from build123d import *

# Parameters (mm, degrees)
SKETCH_W        = 65
SKETCH_H        = 42
PAD_DEPTH       = 4.5
SKETCH001_W     = 2
SKETCH001_H     = 2
POCKET_DEPTH    = 1.5
SKETCH002_W     = 2
SKETCH002_H     = 3
POCKET001_DEPTH = 0.8
SKETCH003_W     = 59
SKETCH003_H     = 35
POCKET002_DEPTH = 3.9
SKETCH004_W     = 2
SKETCH004_H     = 0.4
POCKET003_DEPTH = 5


with BuildPart() as part:
    # Sketch → Pad (new body)
    with BuildSketch(Plane.XY):
        with Locations((-32.5, 0)):
            Rectangle(SKETCH_W, SKETCH_H)
    extrude(amount=-PAD_DEPTH)

    # Sketch001 → Pocket (cut)
    with BuildSketch(Plane.YZ):
        with Locations((-20, -1)):
            Rectangle(SKETCH001_W, SKETCH001_H)
        with Locations((20, -1)):
            Rectangle(SKETCH001_W, SKETCH001_H)
    extrude(amount=-POCKET_DEPTH, mode=Mode.SUBTRACT)

    # Sketch002 → Pocket001 (cut)
    with BuildSketch(Plane.YZ):
        with Locations((-16, -2.2)):
            Rectangle(SKETCH002_W, SKETCH002_H)
        with Locations((-10.8, -2.2)):
            Rectangle(SKETCH002_W, SKETCH002_H)
    extrude(amount=-POCKET001_DEPTH, mode=Mode.SUBTRACT)

    # Sketch003 → Pocket002 (cut)
    with BuildSketch(Plane.XY):
        with Locations((-32.5, 0)):
            Rectangle(SKETCH003_W, SKETCH003_H)
    extrude(amount=-POCKET002_DEPTH, mode=Mode.SUBTRACT)

    # Sketch004 → Pocket003 (cut)
    with BuildSketch(Plane.YZ):
        with Locations((-16, -0.9)):
            Rectangle(SKETCH004_W, SKETCH004_H)
        with Locations((-16, -3.5)):
            Rectangle(SKETCH004_W, SKETCH004_H)
        with Locations((-10.8, -0.9)):
            Rectangle(SKETCH004_W, SKETCH004_H)
        with Locations((-10.8, -3.5)):
            Rectangle(SKETCH004_W, SKETCH004_H)
    extrude(amount=-POCKET003_DEPTH, mode=Mode.SUBTRACT)


solid = part.part
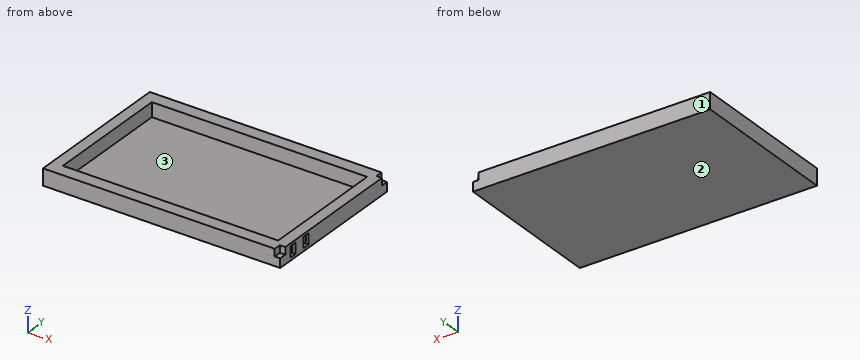
Could you check a few things on this model? Use its own coordinates, in mm. Face numbers are marked on the shaded views. Give positions to 0.01 mm unless a question says otherwise; leave off trailing zeros. Order: outer loops, then holes, each group sorted by start corner. A loop starts at its lowest first (then second) coordinate and runs counter-clockwise, first axis right, second up.
1. Thinking about a two-plate mould opening in Y: for the marked faces 1, 2 and 3, which applies, +Y half, -Y half, draft (parallel to the pull), parting line (faces both ways), or undercut?
Answers below:
face 1: +Y half
face 2: draft
face 3: undercut
2. Suppose I cut it at D-D (y = 10). Write out the boundary of the cut face in (x, z), plus the area to 3 significant figures.
Answers below:
outline: (-65, -4.5) - (0, -4.5) - (0, 0) - (-3, 0) - (-3, -3.9) - (-62, -3.9) - (-62, 0) - (-65, 0) - close
area: 62.4 mm2
3. Suppose I cut it at C-C (x = -35.5). Write out the boundary of the cut face in (y, z), plus the area to 3 significant figures.
Answers below:
outline: (-21, -4.5) - (21, -4.5) - (21, 0) - (17.5, 0) - (17.5, -3.9) - (-17.5, -3.9) - (-17.5, 0) - (-21, 0) - close
area: 52.5 mm2
4. I need wall thicknesses on L1, parallel to X at y = 16, z = -3; L2, parallel to Y at x = -43.5, z = -1.4; L3, parallel to Z at x = -14, y = -16.5. Which ranges of each line are inside material? Lowest first, please.
Answers below:
L1: x = -65 to -62, -3 to 0
L2: y = -21 to -17.5, 17.5 to 21
L3: z = -4.5 to -3.9
5. Suppose I cut it at A-A (z = -2.65). Write out the boundary of the cut face in (x, y), plus the area to 3 significant figures.
Answers below:
outline: (-65, -21) - (0, -21) - (0, -17) - (-0.8, -17) - (-0.8, -15) - (0, -15) - (0, -11.8) - (-0.8, -11.8) - (-0.8, -9.8) - (0, -9.8) - (0, 21) - (-65, 21) - close; hole (-62, -17.5) - (-3, -17.5) - (-3, 17.5) - (-62, 17.5) - close
area: 662 mm2
6. For pin 1 (0.6 mm diameter, centred on y = -16.5, z = -2.5, fed in from +X); pin 2 (1.6 mm diameter, centred on x = -0.5, z = -1, fed in from +Y); pin 3 (5 mm diameter, centred on x = -55.5, y = -11, fed in from +Z), each with a flat end and sliding along its axis, tell me the tip position at first contact or that it passes through.
Answers below:
pin 1: stops at x = -0.8
pin 2: stops at y = 19
pin 3: stops at z = -3.9
7. Suppose I cut it at B-B (y = -11). Write out the boundary of the cut face in (x, z), plus the area to 3 significant figures.
Answers below:
outline: (-65, -4.5) - (0, -4.5) - (0, -3.7) - (-3, -3.7) - (-3, -3.9) - (-62, -3.9) - (-62, 0) - (-65, 0) - close; (-3, -3.3) - (-0.8, -3.3) - (-0.8, -1.1) - (-3, -1.1) - close; (-3, -0.7) - (0, -0.7) - (0, 0) - (-3, 0) - close
area: 58.2 mm2
